Source: CAD feature listing. Evaluate the final solid. Frame: model axes, mm. Coordinates: 2 decimals unless noted, no trailing zeros. Write each loop counter-clockwise with the first axis right and the second up, starting at its lowest first coordinate (ties: lowest second). Pieces come first, ordered by that corner, then holes. Notation, with made-up numbers: (54.25, 64) - (95.25, 64) arc R29 ccw to (95.25, 90) - close; hole circle Ø3 at (-22, 33.5). An arc over 180 degrees is marked (long way). One line per item, written item: value.
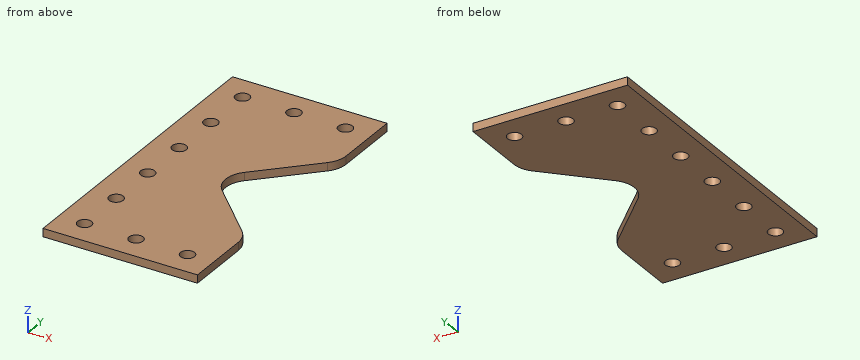
from build123d import *

# Parameters (mm, degrees)
BOSS_EXTRUDE1_DEPTH  = 3.175
M5_CLEARANCE_HOLE1_D = 5.5
LPATTERN1_COUNT      = 3
LPATTERN1_PITCH      = 20
LPATTERN2_COUNT      = 6
LPATTERN2_PITCH      = 20
FILLET2_R            = 10
LPATTERN3_COPY_1_D   = 5.5
LPATTERN3_COPY_2_D   = 5.5
LPATTERN3_COPY_3_D   = 5.5


with BuildPart() as part:
    # Sketch1 → Boss-Extrude1 (new body)
    with BuildSketch(Plane.XY):
        Polygon((0, 0), (0, 120), (60, 120), (60, 90), (30, 60), (60, 30), (60, 0), align=None)
    extrude(amount=BOSS_EXTRUDE1_DEPTH)

    # M5 Clearance Hole1 (through all)
    with Locations(Plane(origin=(10, 10, 3.175), x_dir=(1, 0, 0), z_dir=(0, 0, 1))):
        with Locations((0, 0)):
            m5_clearance_hole1 = Hole(M5_CLEARANCE_HOLE1_D / 2)

    # LPattern1: M5 Clearance Hole1 ×3
    with Locations(*[(i * LPATTERN1_PITCH, 0, 0) for i in range(1, LPATTERN1_COUNT)]):
        add(m5_clearance_hole1, mode=Mode.SUBTRACT)

    # LPattern2: M5 Clearance Hole1 ×6
    with Locations(*[(0, i * LPATTERN2_PITCH, 0) for i in range(1, LPATTERN2_COUNT)]):
        add(m5_clearance_hole1, mode=Mode.SUBTRACT)

    # Fillet2
    fillet2_edges = [part.edges().sort_by_distance(p)[0] for p in [
        (60, 90, 1.5875),
        (30, 60, 1.5875),
        (60, 30, 1.5875),
    ]]
    fillet(fillet2_edges, radius=FILLET2_R)

    # LPattern3 copy 1 (through all)
    with Locations(Plane(origin=(30, 110, 3.175), x_dir=(1, 0, 0), z_dir=(0, 0, 1))):
        with Locations((0, 0)):
            Hole(LPATTERN3_COPY_1_D / 2)

    # LPattern3 copy 2 (through all)
    with Locations(Plane(origin=(50, 110, 3.175), x_dir=(1, 0, 0), z_dir=(0, 0, 1))):
        with Locations((0, 0)):
            Hole(LPATTERN3_COPY_2_D / 2)

    # LPattern3 copy 3 (through all)
    with Locations(Plane(origin=(10, 110, 3.175), x_dir=(1, 0, 0), z_dir=(0, 0, 1))):
        with Locations((0, 0)):
            Hole(LPATTERN3_COPY_3_D / 2)


solid = part.part
1) Section query C-C on z = 1.5. State how many separate pieces and enclosed holes the cut face has, then the cut area to 3 significant figures.
Values found:
separate pieces: 1
enclosed holes: 10
area: 6,080 mm2
2) Section query B-B on y = 110. Output: boundary loops of the cut face in (x, z) (3 decimals).
Values found:
outline: (0, 0) - (7.25, 0) - (7.25, 3.175) - (0, 3.175) - close; (12.75, 0) - (27.25, 0) - (27.25, 3.175) - (12.75, 3.175) - close; (32.75, 0) - (47.25, 0) - (47.25, 3.175) - (32.75, 3.175) - close; (52.75, 0) - (60, 0) - (60, 3.175) - (52.75, 3.175) - close
3) Material intervals for line 1 (Y direction, x = 30, z = 1.3); line 2 (X direction, y = 111.5, z = 2); line 3 (Y direction, x = 35.5, z = 0.6), sorted ascending.
Values found:
line 1: 0 to 7.25, 12.75 to 107.25, 112.75 to 120
line 2: 0 to 7.7, 12.3 to 27.7, 32.3 to 47.7, 52.3 to 60
line 3: 0 to 54.97, 65.03 to 120
4) Section query A-A on x = 30. Output: boundary loops of the cut face in (y, z) (3 decimals).
Values found:
outline: (0, 0) - (7.25, 0) - (7.25, 3.175) - (0, 3.175) - close; (12.75, 0) - (107.25, 0) - (107.25, 3.175) - (12.75, 3.175) - close; (112.75, 0) - (120, 0) - (120, 3.175) - (112.75, 3.175) - close
5) Section query D-D on y = 50. Output: boundary loops of the cut face in (x, z) (3 decimals), then the cut area to 3 significant figures.
Values found:
outline: (0, 0) - (7.25, 0) - (7.25, 3.175) - (0, 3.175) - close; (12.75, 0) - (40, 0) - (40, 3.175) - (12.75, 3.175) - close
area: 110 mm2
